from build123d import *

# Parameters (mm, degrees)
F3_DEPTH = 5
F5_D     = 3.3
F6_R     = 4.5
F7_DEPTH = 5
F8_R     = 57.5
F9_DEPTH = 35


with BuildPart() as f3:
    # F2 (on Top) → F3 (new body)
    with BuildSketch(Plane.XY):
        with BuildLine():
            ThreePointArc((-39.507660736, 48.4292756829), (-31.25, 54.1265877365), (-22.1871526603, 58.4292756829))
            Line((-22.1871526603, 58.4292756829), (-37.8397459622, 85.540362552))
            ThreePointArc((-37.8397459622, 85.540362552), (-51.5, 89.2006165898), (-55.1602540378, 75.540362552))
            Line((-55.1602540378, 75.540362552), (-39.507660736, 48.4292756829))
        make_face()
        with BuildLine():
            ThreePointArc((61.6948133963, -10), (62.2983781381, -5.0161819511), (62.5, 0))
            ThreePointArc((62.5, 0), (62.2983781381, 5.0161819511), (61.6948133963, 10))
            ThreePointArc((61.6948133963, 10), (31.25, 54.1265877365), (-22.1871526603, 58.4292756829))
            ThreePointArc((-22.1871526603, 58.4292756829), (-31.25, 54.1265877365), (-39.507660736, 48.4292756829))
            ThreePointArc((-39.507660736, 48.4292756829), (-62.5, 0), (-39.507660736, -48.4292756829))
            ThreePointArc((-39.507660736, -48.4292756829), (-31.25, -54.1265877365), (-22.1871526603, -58.4292756829))
            ThreePointArc((-22.1871526603, -58.4292756829), (31.25, -54.1265877365), (61.6948133963, -10))
        make_face()
        with BuildLine():
            ThreePointArc((61.6948133963, 10), (62.2983781381, 5.0161819511), (62.5, 0))
            ThreePointArc((62.5, 0), (62.2983781381, -5.0161819511), (61.6948133963, -10))
            Line((61.6948133963, -10), (93, -10))
            ThreePointArc((93, -10), (103, 0), (93, 10))
            Line((93, 10), (61.6948133963, 10))
        make_face()
        with BuildLine():
            Line((-37.8397459622, -85.540362552), (-22.1871526603, -58.4292756829))
            ThreePointArc((-22.1871526603, -58.4292756829), (-31.25, -54.1265877365), (-39.507660736, -48.4292756829))
            Line((-39.507660736, -48.4292756829), (-55.1602540378, -75.540362552))
            ThreePointArc((-55.1602540378, -75.540362552), (-51.5, -89.2006165898), (-37.8397459622, -85.540362552))
        make_face()
    extrude(amount=F3_DEPTH)

    # F5 (through all)
    with Locations(Plane.XY.offset(5)):
        with Locations((-46.5, 80.540362552), (93, 0), (-46.5, -80.540362552)):
            Hole(F5_D / 2)

    # F6 (on face) → F7 (join)
    with BuildSketch(Plane(origin=(0, 0, 0), x_dir=(1, 0, 0), z_dir=(0, 0, -1))):
        Circle(F6_R)
    extrude(amount=F7_DEPTH)

    # F8 (on face) → F9 (join)
    with BuildSketch(Plane.XY.offset(5)):
        with BuildLine():
            ThreePointArc((61.6948133963, -10), (62.2983781381, -5.0161819511), (62.5, 0))
            ThreePointArc((62.5, 0), (62.2983781381, 5.0161819511), (61.6948133963, 10))
            ThreePointArc((61.6948133963, 10), (31.25, 54.1265877365), (-22.1871526603, 58.4292756829))
            ThreePointArc((-22.1871526603, 58.4292756829), (-31.25, 54.1265877365), (-39.507660736, 48.4292756829))
            ThreePointArc((-39.507660736, 48.4292756829), (-62.5, 0), (-39.507660736, -48.4292756829))
            ThreePointArc((-39.507660736, -48.4292756829), (-31.25, -54.1265877365), (-22.1871526603, -58.4292756829))
            ThreePointArc((-22.1871526603, -58.4292756829), (31.25, -54.1265877365), (61.6948133963, -10))
        make_face()
        Circle(F8_R, mode=Mode.SUBTRACT)
    extrude(amount=F9_DEPTH)


solid = f3.part
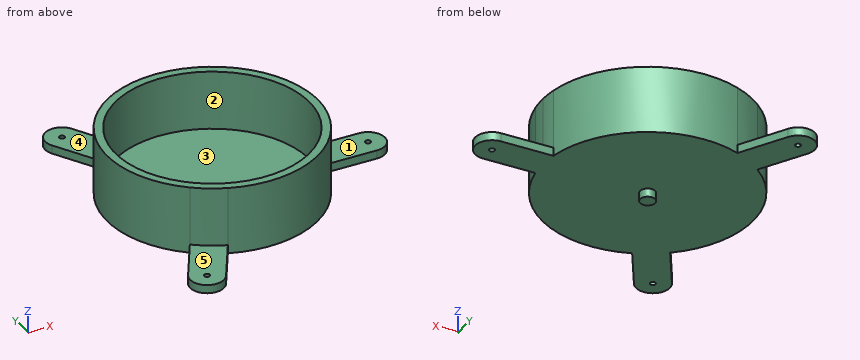
Design review of the part built by this model. Coordinates are the model's own, in mm. Face numbers are marked on the shaded views. A direction names the side the tool comes from. Round coordinates to 2 decimals unless told otherwise and drop trailing zeros. Loops run counter-clockwise (first coordinate to the right, second up) from the corner with the lowest first, then second, coordinate; pieces in that order, holes last. Notation, with made-up numbers: (-20.5, 53.5) -> (27.5, 53.5) arc R27 cw to (27.5, 91.5) -> close; hole circle Ø7 at (33.5, 80.25). An arc over 180 degrees is marked (long way). Use one line per item in the form item = value. Start each with the question number.
Q1. Draft analysis for pull direction X (two halves, no side actions). For the marked faces 1 and 2, state which applies: +X half, -X half, draft (parallel to the pull), parting line (faces both ways), or undercut.
Q2. Wall thickness on line 1 along Y through (x, z) = (93, 2); line 2 along Y through (x, z) = (-46, 3); line 3 along Y through (x, z) = (-46.5, 4): over which ranges is each line inside the solid? List them lowest first. Write a range as [from, to].
Q3. Machinability: for the marked faces 3, 4 and 5, which of the approach directions +Z, -Z, +X, -X, +Y, -Y give a long, thin tool a straight path to every point of the face, cutting with its end or side? Answer none if there is none.
Q4. We need section C-C on y = -18.5. Give the boundary of the cut face in (x, z), then the cut area to 3 significant figures.
Q5. We need section B-B on x = 0. Give the boundary of the cut face in (y, z).
Q6. For pin 1 Ø6 at (x, y) = (89.5, 0) entering from +Z; pin 2 Ø4 at (x, z) = (80.5, 3.5) entering from +Y; pin 3 Ø3 at (x, y) = (35, -32) entering from -Z, all flat-tipped, find the tip position at first contact; note any pin that passes through.
Q7. We need section D-D on x = 33. Give the boundary of the cut face in (y, z), then the cut area to 3 significant figures.
Q8. We need section A-A on z = 8. Give the boundary of the cut face in (x, y).
Calculated:
q1.face_1 = draft
q1.face_2 = undercut
q2.line_1 = [-10, -1.65], [1.65, 10]
q2.line_2 = [-90.53, -82.11], [-78.97, -59.67], [-42.31, 42.31], [59.67, 78.97], [82.11, 90.53]
q2.line_3 = [-90.54, -82.19], [-78.89, -60.54], [-41.76, 41.76], [60.54, 78.89], [82.19, 90.54]
q3.face_3 = +Z
q3.face_4 = +Z, -X, +Y
q3.face_5 = +Z, -X, -Y
q4.outline = (-59.7, 0) -> (59.7, 0) -> (59.7, 40) -> (54.44, 40) -> (54.44, 5) -> (-54.44, 5) -> (-54.44, 40) -> (-59.7, 40) -> close
q4.area = 965 mm²
q5.outline = (-62.5, 0) -> (-4.5, 0) -> (-4.5, -5) -> (4.5, -5) -> (4.5, 0) -> (62.5, 0) -> (62.5, 40) -> (57.5, 40) -> (57.5, 5) -> (-57.5, 5) -> (-57.5, 40) -> (-62.5, 40) -> close
q6.pin_1 = 5
q6.pin_2 = 10
q6.pin_3 = 0
q7.outline = (-53.08, 0) -> (53.08, 0) -> (53.08, 40) -> (47.09, 40) -> (47.09, 5) -> (-47.09, 5) -> (-47.09, 40) -> (-53.08, 40) -> close
q7.area = 950 mm²
q8.outline = circle Ø125 at (0, 0); hole circle Ø115 at (0, 0)
